from build123d import *

# Parameters (mm, degrees)
EXTRUDE_1_DEPTH     = 20
SKETCH_2_R          = 2.4
CUT_EXTRUDE_1_DEPTH = 15
FILLET_1_R          = 1


with BuildPart() as part:
    # 草图1 → 凸台-拉伸1 (new body)
    with BuildSketch(Plane.XY):
        Polygon((0, 20), (0, 0), (10, 0), (10, 3), (3, 3), (3, 20), align=None)
    extrude(amount=EXTRUDE_1_DEPTH)

    # 草图2 → 切除-拉伸1 (cut)
    with BuildSketch(Plane.ZY):
        with Locations(Location((10, 12.5, 0), (0, 0, 270))):
            Circle(SKETCH_2_R)
    extrude(amount=-CUT_EXTRUDE_1_DEPTH, mode=Mode.SUBTRACT)

    # 圆角1
    fillet_1_edges = [part.edges().sort_by_distance(p)[0] for p in [
        (3, 20, 10),
        (3, 3, 10),
        (10, 3, 10),
    ]]
    fillet(fillet_1_edges, radius=FILLET_1_R)


solid = part.part
Geometry check sheet. Reference: the model listing, model coordinates, mm. A direction names the side the tool comes from. Give positions to 0.01 mm unless a question says otherwise; leave off trailing zeros. Order: outer loops, then holes, each group sorted by start corner. A loop starts at its lowest first (then second) coordinate and runs counter-clockwise, first axis right, second up. Notation, with made-up numbers: (73.5, 46) - (120.5, 46) arc R29 cw to (120.5, 79) - close; hole circle Ø3 at (-12.5, 61). An arc over 180 degrees is marked (long way). Answer as a JSON object with one key per item and string values.
(1) Tool access check on faces 4 (the flat face through (0, 8, 10)), 5 (the flat face through (7, 3, 10)). Record the directions out of +Z, -Z, +X, -X, +Y, -Y that give a thin tool (end or side, any length) a straight path to the whole face; none if there is none.
Report:
{"face 4": "+Z, -Z, -X, +Y, -Y", "face 5": "+Z, -Z, +X, +Y"}
(2) Material ranges on line 1 (Z direction, x = 2.45, y = 12.5); line 2 (X direction, y = 9.75, z = 1); line 3 (Y direction, x = 2.5, z = 10.75), recorded low to high.
Report:
{"line 1": "0 to 7.6, 12.4 to 20", "line 2": "0 to 3", "line 3": "0 to 10.22, 14.78 to 19.87"}
(3) Draft check along Z on faces 1 (the cylindrical face through (1.48, 12.81, 12.38)), 2 (the flat face through (2.7, 7.9, 0)), 3 (the flat face through (10, 1, 10)). Enter one of: released by +Z, released by -Z, zero draft, split by the parting line, or undercut.
Report:
{"face 1": "undercut", "face 2": "released by -Z", "face 3": "zero draft"}
(4) Depth check by flat-ended pin: pin 1 Ø1.5 at (y, z) = (15, 5) entering from +X; pin 2 Ø3 at (x, z) = (4, 5.5) entering from +Y; pin 3 Ø2.5 at (x, z) = (5.5, 5.5) entering from +Y. Enter the tip coordinate at first touch or a pass-through.
Report:
{"pin 1": "x = 3", "pin 2": "y = 19.87", "pin 3": "y = 3"}
(5) Cross-section at A-A (y = 12.5). Record the cut outline in (x, z).
Report:
{"outline": "(0, 0) - (3, 0) - (3, 7.6) - (0, 7.6) - close; (0, 12.4) - (3, 12.4) - (3, 20) - (0, 20) - close"}
(6) Cross-section at D-D (z = 17.25). Record the cut outline in (x, y).
Report:
{"outline": "(0, 0) - (10, 0) - (10, 2) arc R1 ccw to (9, 3) - (4, 3) arc R1 cw to (3, 4) - (3, 19) arc R1 ccw to (2, 20) - (0, 20) - close"}
(7) Cross-section at C-C (x = 1). Record the cut outline in (y, z).
Report:
{"outline": "(0, 0) - (20, 0) - (20, 20) - (0, 20) - close; hole circle Ø4.8 at (12.5, 10)"}
(8) Cross-section at B-B (z = 10). Record the cut outline in (x, y), then the cut area to 3 significant figures.
Report:
{"outline": "(0, 0) - (10, 0) - (10, 2) arc R1 ccw to (9, 3) - (4, 3) arc R1 cw to (3, 4) - (3, 10.1) - (0, 10.1) - close; (0, 14.9) - (3, 14.9) - (3, 19) arc R1 ccw to (2, 20) - (0, 20) - close", "area": "66.4 mm^2"}
